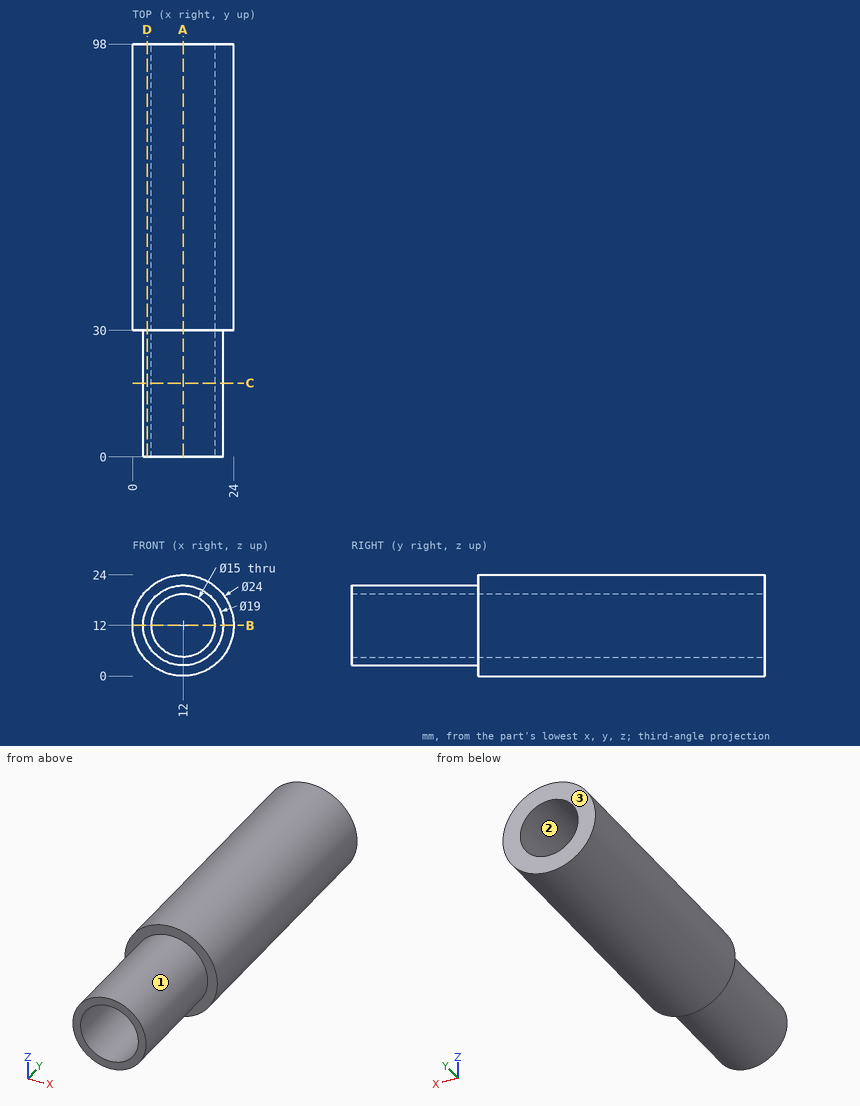
For this review, use the dimensioned drawing (mm, ordinates from the lowest corner) and the shaded views. Coordinates: 2 decimals unless noted, no trailing zeros. Write each loop counter-clockwise with the first axis right and the second up, starting at its lowest first coordinate (ties: lowest second). Pieces come first, ordered by that corner, then holes. Notation, with made-up numbers: (79, 34) -> (121, 34) arc R19 ccw to (121, 55) -> close; hole circle Ø9 at (21, 80). An arc over 180 degrees is marked (long way). Put each result on its own line as item: value.
Q1. Wall thickness on L1, parallel to X at y = 22.5, z = 12; L2, parallel to X at y = 53.5, z = 12: over which ranges is each line inside the solid? List them lowest first.
From the geometry:
L1: x = 2.5 to 4.5, 19.5 to 21.5
L2: x = 0 to 4.5, 19.5 to 24
Q2. The part is to be moulded in two halves that separate along Z. For the marked faces 1, 2 and 3, say which applies: +Z half, -Z half, draft (parallel to the pull), parting line (faces both ways), or undercut.
From the geometry:
face 1: parting line
face 2: undercut
face 3: draft
Q3. Take a section at B-B, the plane z = 12. State the section outline as (x, y) points.
From the geometry:
outline: (0, 30) -> (2.5, 30) -> (2.5, 0) -> (4.5, 0) -> (4.5, 98) -> (0, 98) -> close; (19.5, 0) -> (21.5, 0) -> (21.5, 30) -> (24, 30) -> (24, 98) -> (19.5, 98) -> close
Q4. Take a section at D-D, the plane x = 3.5. State the section outline as (y, z) points, then the cut area to 3 significant figures.
From the geometry:
outline: (0, 7.76) -> (30, 7.76) -> (30, 3.53) -> (98, 3.53) -> (98, 20.47) -> (30, 20.47) -> (30, 16.24) -> (0, 16.24) -> close
area: 1,410 mm2
Q5. Take a section at C-C, the plane y = 17.5. State the section outline as (x, z) points.
From the geometry:
outline: circle Ø19 at (12, 12); hole circle Ø15 at (12, 12)
Q6. Take a section at A-A, the plane x = 12. State the section outline as (y, z) points, then the cut area to 3 significant figures.
From the geometry:
outline: (0, 2.5) -> (30, 2.5) -> (30, 0) -> (98, 0) -> (98, 4.5) -> (0, 4.5) -> close; (0, 19.5) -> (98, 19.5) -> (98, 24) -> (30, 24) -> (30, 21.5) -> (0, 21.5) -> close
area: 732 mm2
Q7. Clearance check with flat-ended pins moving along their axes: pin 1 Ø2 at (y, z) = (28, 13) entering from +X; pin 2 Ø4 at (x, z) = (10, 15) entering from +Y; pin 3 Ø1 at (y, z) = (56.5, 15.5) entering from -X; pin 4 Ø5 at (y, z) = (80.5, 6) entering from -X. State where each tip first meets the part, or that it passes through.
From the geometry:
pin 1: stops at x = 21.5
pin 2: passes through
pin 3: stops at x = 0.38
pin 4: stops at x = 0.52
